from build123d import *

# Parameters (mm, degrees)
SKETCH1_W           = 23.89
SKETCH1_H           = 15.84
BOSS_EXTRUDE1_DEPTH = 3.17
SKETCH2_R           = 2.445
BOSS_EXTRUDE2_DEPTH = 1.89
SHELL1_T            = -0.8
SKETCH3_R           = 2.975
SKETCH3_R_2         = 2.83
BOSS_EXTRUDE3_DEPTH = 1.47


with BuildPart() as part:
    # Sketch1 → Boss-Extrude1 (new body)
    with BuildSketch(Plane(origin=(0, 0, 0), x_dir=(1, 0, 0), z_dir=(0, 1, 0))):
        Rectangle(SKETCH1_W, SKETCH1_H)
    extrude(amount=-BOSS_EXTRUDE1_DEPTH)

    # Sketch2 → Boss-Extrude2 (add)
    with BuildSketch(Plane(origin=(0, 0, 0), x_dir=(1, 0, 0), z_dir=(0, 1, 0))):
        with Locations(Location((-7.963333333, 3.96, 0), (0, 0, 90))):
            Circle(SKETCH2_R)
        with Locations(Location((0, 3.96, 0), (0, 0, 90))):
            Circle(SKETCH2_R)
        with Locations(Location((7.963333333, 3.96, 0), (0, 0, 90))):
            Circle(SKETCH2_R)
        with Locations(Location((-7.965, -3.96, 0), (0, 0, 90))):
            Circle(SKETCH2_R)
        with Locations(Location((-0.005, -3.96, 0), (0, 0, 90))):
            Circle(SKETCH2_R)
        with Locations(Location((7.955, -3.96, 0), (0, 0, 90))):
            Circle(SKETCH2_R)
    extrude(amount=BOSS_EXTRUDE2_DEPTH)

    # Shell1
    shell1_openings = [part.faces().sort_by_distance(p)[0] for p in [
        (0, -3.17, 0),
    ]]
    offset(amount=SHELL1_T, openings=shell1_openings, kind=Kind.INTERSECTION)

    # Sketch3 → Boss-Extrude3 (add)
    # profile 1 of 2: a face of its own
    with BuildSketch(Plane.XZ.offset(0.8)):
        with Locations(Location((3.981666667, 0, 0), (0, 0, 90))):
            Circle(SKETCH3_R)
        with Locations(Location((3.981666667, 0, 0), (0, 0, 270))):
            Circle(SKETCH3_R_2, mode=Mode.SUBTRACT)
    # profile 2 of 2: a face of its own
    with BuildSketch(Plane.XZ.offset(0.8)):
        with Locations(Location((-3.981666667, 0, 0), (0, 0, 90))):
            Circle(SKETCH3_R)
        with Locations(Location((-3.981666667, 0, 0), (0, 0, 270))):
            Circle(SKETCH3_R_2, mode=Mode.SUBTRACT)
    extrude(amount=BOSS_EXTRUDE3_DEPTH)


solid = part.part
Here's how the part is built. I have some questions about the finished solid (model axes, mm). A direction names the side the tool comes from. Round coordinates to 2 decimals unless told otherwise and drop trailing zeros. Loops run counter-clockwise (first coordinate to the right, second up) from the corner with the lowest first, then second, coordinate; pieces in that order, holes last.
1. If we section it at B-B on y = -0.4: Write out the boundary of the cut face in (x, z) (3 decimals), plus the area to 3 significant figures.
Answer list:
outline: (-11.945, -7.92) - (11.945, -7.92) - (11.945, 7.92) - (-11.945, 7.92) - close; hole circle Ø3.29 at (-7.965, 3.96); hole circle Ø3.29 at (-7.963, -3.96); hole circle Ø3.29 at (-0.005, 3.96); hole circle Ø3.29 at (0, -3.96); hole circle Ø3.29 at (7.955, 3.96); hole circle Ø3.29 at (7.963, -3.96)
area: 327 mm2
2. We'd pull the mould along X, two halves only. Please class faces 1 (the face through (6.324, 0.132, 4.174)), 2 (the face through (-8, 1.89, -4)): +X half, -X half, draft (parallel to the pull), parting line (faces both ways), or undercut.
Answer list:
face 1: undercut
face 2: draft
3. If I drill on line 1 along X through (y, z) = (-0.1, -3.96) (3 decimals); line 2 along X through (y, z) = (0.7, 3.96); line 3 along Z through (x, y) = (-10, -2.4), over which ranges is the centre line in solid material (lowest first)?
Answer list:
line 1: x = -11.945 to -9.608, -6.318 to -1.645, 1.645 to 6.318, 9.608 to 11.945
line 2: x = -10.41 to -9.61, -6.32 to -5.52, -2.45 to -1.65, 1.64 to 2.44, 5.51 to 6.31, 9.6 to 10.4
line 3: z = -7.92 to -7.12, 7.12 to 7.92
4. Which directions (+Z, -Z, +X, -X, +Y, -Y) give clear straight access to the entire face, cutting with the end or side of a thin tool? Please do faces 3 (the face through (-0.9, -3.17, 7.6)), 4 (the face through (-5.8, 0.9, -5.1)), 5 (the face through (0, 1.09, -4)).
Answer list:
face 3: +Z, -Z, +X, -X, -Y
face 4: +Y
face 5: -Y
5. For P1, Ø3, axis at x = -5.5, z = -0.5, coming from the -Y side; P2, Ø4.5, axis at x = -3.98, z = 0, coming from the +Y side; P3, Ø1.6, axis at x = -8.5, z = -4, coming from the -Y side; P4, Ø6, axis at x = -1, z = -5.5, coming from the -Y side, each with a flat end and sliding along its axis, tell me the tip position at first contact or that it passes through.
Answer list:
P1: stops at y = -2.27
P2: stops at y = 0
P3: stops at y = 1.09
P4: stops at y = -3.17
6. If we section it at C-C on x = 10: Write out the boundary of the cut face in (y, z).
Answer list:
outline: (-3.17, -7.92) - (0, -7.92) - (0, -5.31) - (1.89, -5.31) - (1.89, -2.61) - (0, -2.61) - (0, 2.62) - (1.89, 2.62) - (1.89, 5.3) - (0, 5.3) - (0, 7.92) - (-3.17, 7.92) - (-3.17, 7.12) - (-0.8, 7.12) - (-0.8, -7.12) - (-3.17, -7.12) - close
7. If we section it at D-D on z = 0: Write out the boundary of the cut face in (x, y) (3 decimals).
Answer list:
outline: (-11.945, -3.17) - (-11.145, -3.17) - (-11.145, -0.8) - (-6.957, -0.8) - (-6.957, -2.27) - (-6.812, -2.27) - (-6.812, -0.8) - (-1.152, -0.8) - (-1.152, -2.27) - (-1.007, -2.27) - (-1.007, -0.8) - (1.007, -0.8) - (1.007, -2.27) - (1.152, -2.27) - (1.152, -0.8) - (6.812, -0.8) - (6.812, -2.27) - (6.957, -2.27) - (6.957, -0.8) - (11.145, -0.8) - (11.145, -3.17) - (11.945, -3.17) - (11.945, 0) - (-11.945, 0) - close
